Job drawing, mm, ordinate dimensions from the low corner. One solid piece. Give positions to 0.01 mm unless a question says otherwise; leave off trailing zeros. Order: outer loops, then holes, each group sorted by start corner. A loop starts at its lowest first (then second) coordinate and runs counter-clockwise, first axis right, second up. Notation, with made-up numbers: (34, 39.25) - (71, 39.25) arc R15 ccw to (71, 67.25) - close; hole circle Ø6 at (22.25, 9). An arc over 180 degrees is marked (long way). Use one line per item in the form item = value. Start each with the question number.
1. Band-saw the part on A-A, the plane z = 0.25. List the corners of the cut face in (x, y).
2. Band-saw the part on D-D, the plane x = 9.75. List the corners of the cut face in (y, z), plus the area to 3 significant figures.
3. Band-saw the part on C-C, the plane x = 1.5. List the corners of the cut face in (y, z).
4. Drill centre lines: line 1 (Y direction, x = 21, z = 0.2); line 2 (Z direction, x = 3.5, y = 3.5); line 3 (Y direction, x = 12, z = 0.9). Where is each one in solid material? Low to high.
5. Pin check, flat tip, straight feed: P1, Ø5, axis at x = 17, y = 18.5, coming from the +Z side. Stop position of the tip, or through.
6. Band-saw the part on B-B, the plane y = 9.5. List the corners of the cut face in (x, z).
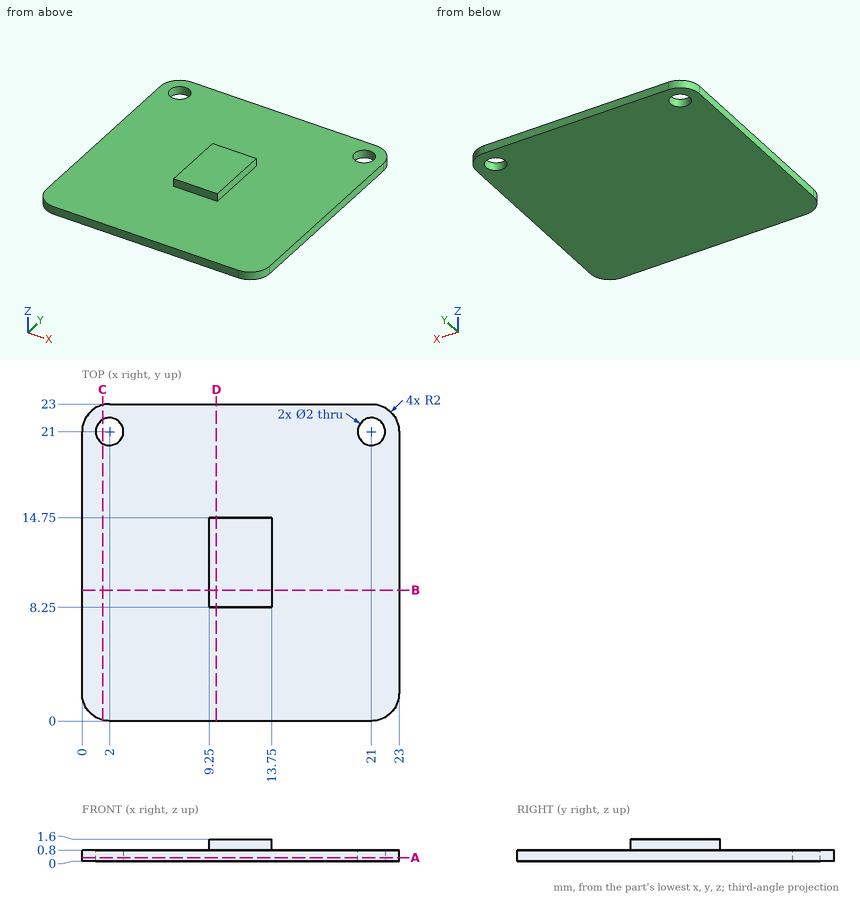
From the geometry:
q1.outline = (0, 2) arc R2 ccw to (2, 0) - (21, 0) arc R2 ccw to (23, 2) - (23, 21) arc R2 ccw to (21, 23) - (2, 23) arc R2 ccw to (0, 21) - close; hole circle Ø2 at (2, 21); hole circle Ø2 at (21, 21)
q2.outline = (0, 0) - (23, 0) - (23, 0.8) - (14.75, 0.8) - (14.75, 1.6) - (8.25, 1.6) - (8.25, 0.8) - (0, 0.8) - close
q2.area = 23.6 mm²
q3.outline = (0.06, 0) - (20.13, 0) - (20.13, 0.8) - (0.06, 0.8) - close; (21.87, 0) - (22.94, 0) - (22.94, 0.8) - (21.87, 0.8) - close
q4.line_1 = 0 to 20, 22 to 23
q4.line_2 = 0 to 0.8
q4.line_3 = 8.25 to 14.75
q5.P1 = 0.8
q6.outline = (0, 0) - (23, 0) - (23, 0.8) - (13.75, 0.8) - (13.75, 1.6) - (9.25, 1.6) - (9.25, 0.8) - (0, 0.8) - close
